The figure shows three views and two pictorial views of one solid part (mm, origin at its lowest corner). Answer the questions. A direction names the side the tool comes from. Coordinates: 2 decimals unless noted, no trailing zeros. Loops run counter-clockwise (first coordinate to the right, second up) from the corner with the lowest first, then second, coordinate; pieces in that order, holes last. Notation, with made-up numbers: M 9.5,19.25 L 64.5,19.25 A20 ccw 64.5,40.25 Z; hole C 11.5,-30 d7. An arc over 180 degrees is marked long. One line per item, written item: value. Start each with the question number.
1. Flat-ended cylindrical pins translate along their axes: pin 1 (3 mm diameter, centred on x = 43, y = 3, fed in from +Z); pin 2 (5 mm diameter, centred on x = 48, y = 6.5, fed in from -Z); pin 3 (1.5 mm diameter, centred on y = 4, z = 34.5, fed in from +X). Find the tip coordinate at first contact, or state that the pin passes through.
2. Consider probe 1 along X at (y, z) = (6.5, 30); probe 2 along X at (y, z) = (0.8, 30); probe 3 along X at (y, z) = (7.25, 54). Determine where each line is inside the solid, lowest interval first.
3. The part is cut by section A-A (x = 54). Write down the section's boundary in (y, z).
4. For the marked faces 1, 2, 3 and 4, determine the directions among +Z, -Z, +X, -X, +Y, -Y from which every point of the face is accessible in a straight line to the end or side of a thin tool.
5. The part is cut by section D-D (y = 1). State how many separate pieces and enclosed holes the cut face has, then the cut area to 3 significant figures.
6. The part is cut by section B-B (z = 30). Write down the section's boundary in (x, y).
7. The part is cut by section C-C (x = 30). Write down the section's boundary in (y, z).
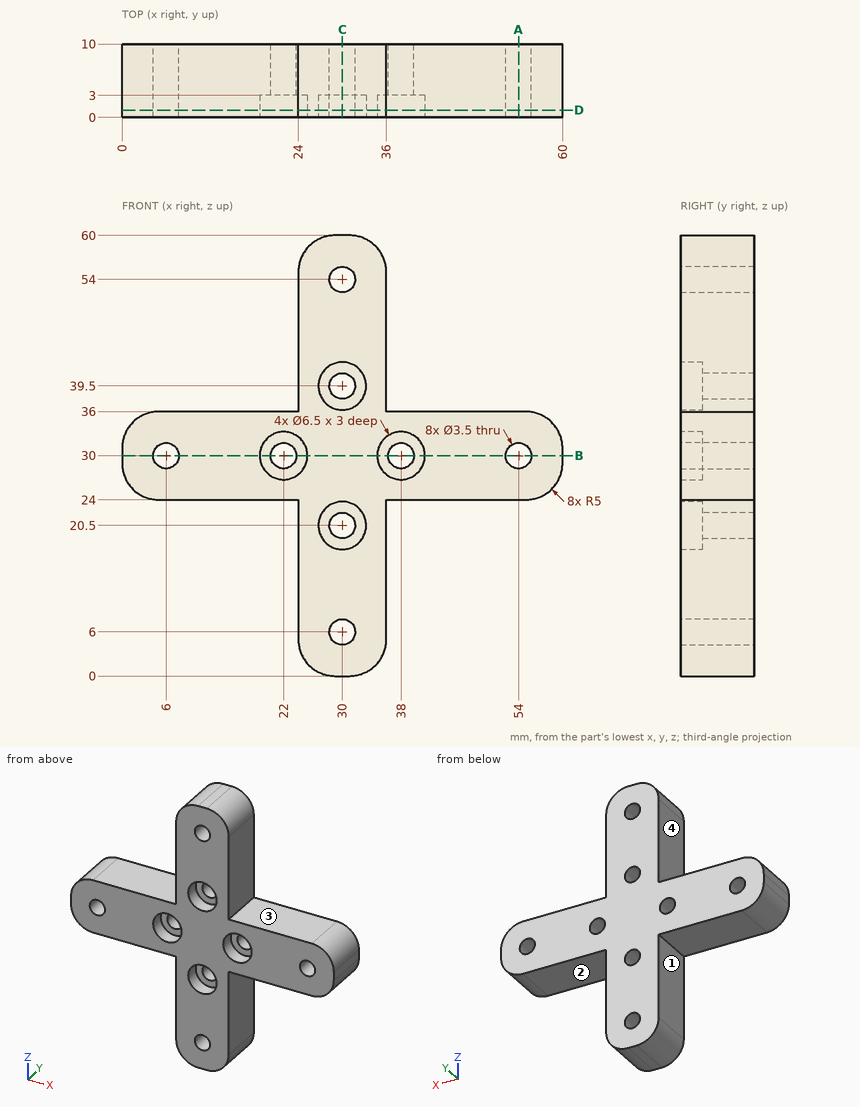
Answer block:
1. pin 1: stops at z = 36
1. pin 2: stops at z = 24
1. pin 3: stops at x = 59.18
2. probe 1: x = 0 to 4.25, 7.75 to 20.25, 23.75 to 36.25, 39.75 to 52.25, 55.75 to 60
2. probe 2: x = 0 to 4.25, 7.75 to 18.75, 25.25 to 34.75, 41.25 to 52.25, 55.75 to 60
2. probe 3: x = 24 to 28.25, 31.75 to 36
3. outline: M 0,24 L 10,24 L 10,28.25 L 0,28.25 Z; M 0,31.75 L 10,31.75 L 10,36 L 0,36 Z
4. face 1: -Z, -X, +Y, -Y
4. face 2: -Z, +X, +Y, -Y
4. face 3: +Z, +X, +Y, -Y
4. face 4: +Z, -X, +Y, -Y
5. separate pieces: 1
5. enclosed holes: 8
5. area: 1,080 mm2
6. outline: M 0,0 L 4.25,0 L 4.25,10 L 0,10 Z; M 7.75,0 L 18.75,0 L 18.75,3 L 20.25,3 L 20.25,10 L 7.75,10 Z; M 23.75,3 L 25.25,3 L 25.25,0 L 34.75,0 L 34.75,3 L 36.25,3 L 36.25,10 L 23.75,10 Z; M 39.75,3 L 41.25,3 L 41.25,0 L 52.25,0 L 52.25,10 L 39.75,10 Z; M 55.75,0 L 60,0 L 60,10 L 55.75,10 Z
7. outline: M 0,0 L 10,0 L 10,4.25 L 0,4.25 Z; M 0,7.75 L 10,7.75 L 10,18.75 L 3,18.75 L 3,17.25 L 0,17.25 Z; M 0,23.75 L 3,23.75 L 3,22.25 L 10,22.25 L 10,37.75 L 3,37.75 L 3,36.25 L 0,36.25 Z; M 0,42.75 L 3,42.75 L 3,41.25 L 10,41.25 L 10,52.25 L 0,52.25 Z; M 0,55.75 L 10,55.75 L 10,60 L 0,60 Z
